For this review, take the finished solid that the model builds, in its own axes (mm). Face numbers are marked on the shaded views. A direction names the side the tool comes from. Round coordinates to 2 decimals unless told otherwise and drop trailing zeros. Write each loop counter-clockwise with the first axis right and the second up, starting at its lowest first coordinate (ties: lowest second). Pieces come first, ordered by that corner, then holes. Notation, with made-up numbers: (-35, 58.5) -> (4, 58.5) arc R33 cw to (4, 86.5) -> close; hole circle Ø5 at (24, -35). An arc over 180 degrees is marked (long way). Write each question's results on one line, items separated by ' | '. Start each with the question number.
Item 1: Tool access review of the marked faces 1 and 2: name each direction out of +Z, -Z, +X, -X, +Y, -Y from which nothing blocks a thin tool from reaching the whole face with its end or side.
Item 2: The part is to be moulded in two halves that separate along Y. For the marked faces 3, 4, 5 and 6, say which applies: +Y half, -Y half, draft (parallel to the pull), parting line (faces both ways), or undercut.
Item 3: Add section D-D (x = -0.5). State the section outline as (y, z) points, plus the area to 3 significant figures.
Item 4: Add section B-B (y = 0). State the section outline as (x, z) points, plus the area to 4 significant figures.
Item 5: Clearance check with flat-ended pins moving along their axes: pin 1 (1.5 mm diameter, centred on x = 5, z = 9, fed in from +Y); pin 2 (4 mm diameter, centred on x = 1.5, z = 6.5, fed in from -Y); pin 3 (2 mm diameter, centred on x = 3.5, y = 15, fed in from -Z). State where each tip first meets the part, or that it passes through.
Item 6: To check wall thickness, follow line 1 along Y through (x, z) = (-1.65, 0); line 2 along Y through (x, z) = (4.5, 0); line 3 along Z through (x, y) = (-3, -14.5). State the ranges of each line that lie inside material, in increasing order.
Item 7: Add section A-A (z = 0). State the section outline as (x, y) points.
Item 8: Add section C-C (x = 4.5). State the section outline as (y, z) points, plus the area to 3 significant figures.
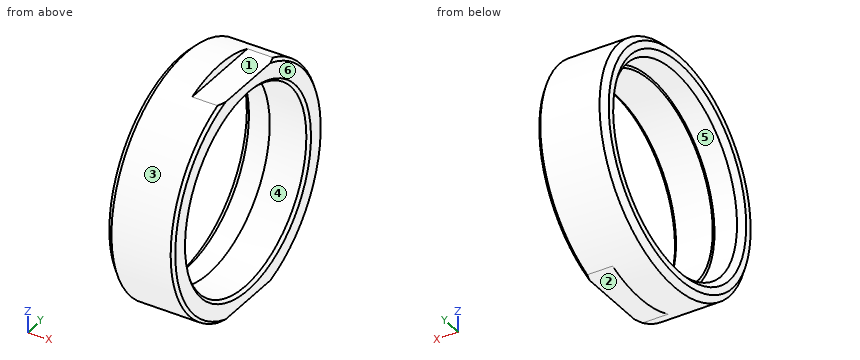
from build123d import *

# Parameters (mm, degrees)
ESQUISSE2_W             = 6.395173454
ESQUISSE2_H             = 30.286576169
ENL_V_MAT_EXTRU_1_DEPTH = 5


with BuildPart() as part:
    # Esquisse1 → R_volution1 (revolve)
    with BuildSketch(Plane.XY, mode=Mode.PRIVATE) as r_volution1_sk:
        Polygon((0, 17.75), (-4, 17.75), (-5, 18.75), (-5, 20), (-4, 21), (6.5, 21), (7, 20.5), (7, 17.75), (6.5, 17.25), (0, 17.25), align=None)
    revolve(r_volution1_sk.sketch.rotate(Axis((-33.075824176, 0, 0), (1, 0, 0)), 90), axis=Axis((-33.075824176, 0, 0), (1, 0, 0)))

    # Esquisse2 → Enl_v. mat.-Extru.1 (cut)
    with BuildSketch(Plane(origin=(7, 0, 0), x_dir=(0, 0, -1), z_dir=(1, 0, 0))):
        with Locations((-22.697586727, -0.422322776)):
            Rectangle(ESQUISSE2_W, ESQUISSE2_H)
        with Locations((22.697586727, -0.422322776)):
            Rectangle(ESQUISSE2_W, ESQUISSE2_H)
    extrude(amount=-ENL_V_MAT_EXTRU_1_DEPTH, mode=Mode.SUBTRACT)


solid = part.part
Responses:
1) face 1: +Z, +X, +Y, -Y | face 2: -Z, +X, +Y, -Y
2) face 3: parting line | face 4: undercut | face 5: undercut | face 6: draft
3) outline: circle Ø42 at (0, 0); hole circle Ø35.5 at (0, 0) | area: 396 mm^2
4) outline: (-5, -20) -> (-4, -21) -> (2, -21) -> (2, -19.5) -> (7, -19.5) -> (7, -17.75) -> (6.5, -17.25) -> (0, -17.25) -> (0, -17.75) -> (-4, -17.75) -> (-5, -18.75) -> close; (-5, 18.75) -> (-4, 17.75) -> (0, 17.75) -> (0, 17.25) -> (6.5, 17.25) -> (7, 17.75) -> (7, 19.5) -> (2, 19.5) -> (2, 21) -> (-4, 21) -> (-5, 20) -> close | area: 67.75 mm^2
5) pin 1: stops at y = 19.31 | pin 2: stops at y = -20.51 | pin 3: stops at z = -15.65
6) line 1: y = -21 to -17.75, 17.75 to 21 | line 2: y = -21 to -17.25, 17.25 to 21 | line 3: z = -15.19 to -10.24, 10.24 to 15.19
7) outline: (-5, -20) -> (-4, -21) -> (6.5, -21) -> (7, -20.5) -> (7, -17.75) -> (6.5, -17.25) -> (0, -17.25) -> (0, -17.75) -> (-4, -17.75) -> (-5, -18.75) -> close; (-5, 18.75) -> (-4, 17.75) -> (0, 17.75) -> (0, 17.25) -> (6.5, 17.25) -> (7, 17.75) -> (7, 20.5) -> (6.5, 21) -> (-4, 21) -> (-5, 20) -> close
8) outline: (-7.79, -19.5) -> (7.79, -19.5) arc R21 ccw to (7.79, 19.5) -> (-7.79, 19.5) arc R21 ccw to start; hole circle Ø34.5 at (0, 0) | area: 419 mm^2
